Build history of the part. All positions in model axes, mm. Give positions to 0.01 mm unless a question says otherwise; leave off trailing zeros. Order: outer loops, then holes, each group sorted by start corner. A loop starts at its lowest first (then second) coordinate and runs counter-clockwise, first axis right, second up. Notation, with made-up numbers: M -21,52.25 L 37,52.25 A24 ccw 37,82.25 Z; hole C 62.5,66 d10. An arc over 180 degrees is marked long. One line per item, written item: value.
from build123d import *

# Parameters (mm, degrees)
F0_W     = 49.954958
F0_H     = 58.300882
F1_DEPTH = 12.7
F2_R     = 12.587568
F3_DEPTH = 25.401


with BuildPart() as f1:
    # F0 (on Top) → F1 (new body, symmetric)
    with BuildSketch(Plane.XY):
        with Locations((-102.361765, 17.77092)):
            Rectangle(F0_W, F0_H)
    extrude(amount=F1_DEPTH, both=True)

    # F2 (on face) → F3 (cut, through all)
    with BuildSketch(Plane.XY.offset(12.7)):
        with Locations((-103.024021, 16.906289)):
            Circle(F2_R)
    extrude(amount=-F3_DEPTH, mode=Mode.SUBTRACT)

    # F4 (on face) → F5 (revolve)
    with BuildSketch(Plane.XY.offset(12.7)):
        Polygon((-113.443017, 34.847543), (-113.443017, 38.281992), (-115.650638, 40.912932), (-119.03291, 41.509318), (-122.00723, 39.792094), (-123.181881, 36.564767), (-122.00723, 33.337441), (-119.03291, 31.620217), (-115.650638, 32.216602), align=None)
    revolve(axis=Axis((-77.384286, 17.77092, 12.7), (0, -1, 0)))


solid = f1.part
1) Saw through at C-C, the plane y = 19.5. Write the cut outline in (x, z), then the cut area to 3 significant figures.
Check values:
outline: M -127.34,-12.7 L -115.34,-12.7 L -115.34,12.7 L -127.34,12.7 Z; M -90.71,-12.7 L -77.38,-12.7 L -77.38,12.7 L -90.71,12.7 Z
area: 643 mm^2
2) Saw through at B-B, the plane z = 4. Give the number of separate pieces and of enclosed holes in the cut face, then the cut area to 3 significant figures.
Check values:
separate pieces: 2
enclosed holes: 1
area: 2,490 mm^2
3) Drill centre lines: probe 1 along Z at (x, y) = (-90.5, 35); probe 2 along Z at (x, y) = (-100, 34); probe 3 along X at (y, z) = (39.5, -13.5). Where is each one in solid material? Low to high. Write a range as from..to.
Check values:
probe 1: -30.58..-20.89, -12.7..12.7, 46.29..55.98
probe 2: -26.05..-16.29, -12.7..12.7, 41.69..51.45
probe 3: -113.64..-103.62, -51.14..-41.13
4) Mould opens along Z. For faces 1 (the face through (-103, -11.38, 0)), 2 (the face through (-37.029, 31.704, 23.567)), 3 (the face through (-40.5, 40.95, 23.65)) say: released by +Z, released by -Z, zero draft, split by the parting line, or undercut.
Check values:
face 1: zero draft
face 2: split by the parting line
face 3: undercut
5) Saw through at A-A, the plane y = 13.5. Write the cut outline in (x, z).
Check values:
outline: M -127.34,-12.7 L -115.14,-12.7 L -115.14,12.7 L -127.34,12.7 Z; M -90.91,-12.7 L -77.38,-12.7 L -77.38,12.7 L -90.91,12.7 Z
6) Saw through at D-D, the plane y = -2. Write the cut outline in (x, z).
Check values:
outline: M -127.34,-12.7 L -77.38,-12.7 L -77.38,12.7 L -127.34,12.7 Z
7) Pin check, flat tips, straight feed: pin 1 (4 mm diameter, centred on y = 40.5, z = 12, fed in from +X); pin 2 (25 mm diameter, centred on x = -114, y = 25.5, fed in from +Z); pin 3 (10 mm diameter, centred on y = 30, z = 3.5, fed in from +X). Stop position of each tip, or through.
Check values:
pin 1: x = -32.3
pin 2: z = 48.32
pin 3: x = -32.89
